```python
from build123d import *

# Parameters (mm, degrees)
F0_W     = 35
F0_H     = 15
F0_W_2   = 10
F0_R     = 2
F1_DEPTH = 6
F2_SIZE  = 3
F3_R     = 2
F4_DEPTH = 12
F5_DEPTH = 6
F6_R     = 2
F7_DEPTH = 15.001


with BuildPart() as f1:
    # F0 (on Top) → F1 (new body)
    with BuildSketch(Plane.XY):
        with Locations((22.5, 0)):
            Rectangle(F0_W, F0_H)
        Rectangle(F0_W_2, F0_H)
        Circle(F0_R, mode=Mode.SUBTRACT)
        with Locations((-22.5, 0)):
            Rectangle(F0_W, F0_H)
    extrude(amount=F1_DEPTH)

    # F2
    f2_edges = [f1.edges().sort_by_distance(p)[0] for p in [
        (0, -7.5, 6),
        (-40, 0, 6),
        (40, 0, 6),
        (0, 7.5, 6),
    ]]
    chamfer(f2_edges, length=F2_SIZE)

    # F3 (on face) → F4 (cut)
    with BuildSketch(Plane(origin=(0, 0, 0), x_dir=(1, 0, 0), z_dir=(0, 0, -1))):
        with Locations((-30, 0)):
            Circle(F3_R)
        with Locations((-15, 0)):
            Circle(F3_R)
        with Locations((15, 0)):
            Circle(F3_R)
        with Locations((30, 0)):
            Circle(F3_R)
    extrude(amount=-F4_DEPTH, mode=Mode.SUBTRACT)

    # F0 (on Top) → F5 (join)
    with BuildSketch(Plane.XY):
        Rectangle(F0_W_2, F0_H)
        Circle(F0_R, mode=Mode.SUBTRACT)
    extrude(amount=F5_DEPTH)

    # F6 (on face) → F7 (cut, through all)
    with BuildSketch(Plane.XZ.offset(7.5)):
        with Locations((0, 3)):
            Circle(F6_R)
    extrude(amount=-F7_DEPTH, mode=Mode.SUBTRACT)


solid = f1.part
```
The model under review builds one solid part; all positions refer to its coordinate system, in mm. A direction names the side the tool comes from. Give positions to 0.01 mm unless a question says otherwise; leave off trailing zeros. Write each loop counter-clockwise with the first axis right and the second up, starting at its lowest first coordinate (ties: lowest second). Pieces come first, ordered by that corner, then holes. Notation, with made-up numbers: (1.25, -40) - (6.25, -40) arc R23 cw to (6.25, -8) - close; hole circle Ø10 at (1.5, -32). An arc over 180 degrees is marked (long way). Answer in a Markdown table with one row per item. Add a question column.
1. We need section A-A on x = 0. Write out the cut boundary in (y, z), then the cut area to 3 significant figures.
2. Wall thickness on line 1 along X through (y, z) = (-0.75, 1.4); line 2 along X through (y, z) = (-5, 3); line 3 along X through (y, z) = (0, 3.35): over which ranges is each line inside the solid? List them lowest first. Write a range as [from, to].
3. We need section D-D on z = 4.1. Write out the cut boundary in (x, y).
4. Insertion check: P1, Ø3, axis at y = -5, z = 5, coming from the -X side; P2, Ø2.5, axis at x = 0, z = 3, coming from the -Y side; P3, Ø1.5, axis at y = 6.5, z = 4.5, coming from the +X side; P4, Ø0.9, axis at y = -6, z = 4.5, coming from the +X side. Each pin has a flat end and moves straight along its axis. Give the tip position at first contact, or say it passes through.
5. We need section B-B on x = -30. Write out the cut boundary in (y, z), then the cut area to 3 significant figures.
6. We need section C-C on y = 3.75. Write out the cut boundary in (x, z), then the cut area to 3 significant figures.
7. Draft analysis for pull direction Y (two halves, no side actions). For faces 5 (the cylindrical face through (-1.6, -4.6, 1.8)), 6 (the cylindrical face through (31.908, -0.601, 2.958)), 7 (the flat face through (1, 7.5, 1)), state which applies: +Y half, -Y half, draft (parallel to the pull), parting line (faces both ways), or undercut.
8. Tool access review of faces 1 (the flat face through (-5, 7, 5)), 2 (the cylindrical face through (-2, 0, 5)), 3 (the flat face through (5, 7, 5)), 4 (the flat face through (-22.7, -6, 4.5)): name each direction out of +Z, -Z, +X, -X, +Y, -Y from which nothing blocks a thin tool from reaching the whole face with its end or side.
Ans:
| question | item | result |
|---|---|---|
| 1 | outline | (-7.5, 0) - (-2, 0) - (-2, 1) - (-7.5, 1) - close; (-7.5, 5) - (-2, 5) - (-2, 6) - (-7.5, 6) - close; (2, 0) - (7.5, 0) - (7.5, 1) - (2, 1) - close; (2, 5) - (7.5, 5) - (7.5, 6) - (2, 6) - close |
| 1 | area | 22.0 mm^2 |
| 2 | line 1 | x = [-40, -31.85], [-28.15, -16.85], [-13.15, -1.85], [1.85, 13.15], [16.85, 28.15], [31.85, 40] |
| 2 | line 2 | x = [-40, -2], [2, 40] |
| 2 | line 3 | x = [-39.65, -32], [-28, -17], [-13, -2], [2, 13], [17, 28], [32, 39.65] |
| 3 | outline | (-38.9, -6.4) - (-5, -6.4) - (-5, -7.5) - (-1.67, -7.5) - (-1.67, -1.1) arc R2 cw to (-1.67, 1.1) - (-1.67, 7.5) - (-5, 7.5) - (-5, 6.4) - (-38.9, 6.4) - close; (1.67, -7.5) - (5, -7.5) - (5, -6.4) - (38.9, -6.4) - (38.9, 6.4) - (5, 6.4) - (5, 7.5) - (1.67, 7.5) - (1.67, 1.1) arc R2 cw to (1.67, -1.1) - close; hole circle Ø4 at (-30, 0); hole circle Ø4 at (-15, 0); hole circle Ø4 at (15, 0); hole circle Ø4 at (30, 0) |
| 4 | P1 | stops at x = -39.5 |
| 4 | P2 | passes through |
| 4 | P3 | stops at x = 39.25 |
| 4 | P4 | stops at x = 38.95 |
| 5 | outline | (-7.5, 0) - (-2, 0) - (-2, 6) - (-4.5, 6) - (-7.5, 3) - close; (2, 0) - (7.5, 0) - (7.5, 3) - (4.5, 6) - (2, 6) - close |
| 5 | area | 57.0 mm^2 |
| 6 | outline | (-40, 0) - (40, 0) - (40, 3) - (37, 6) - (-37, 6) - (-40, 3) - close; hole circle Ø4 at (0, 3) |
| 6 | area | 458 mm^2 |
| 7 | face 5 | draft |
| 7 | face 6 | undercut |
| 7 | face 7 | +Y half |
| 8 | face 1 | +Z, -X, +Y |
| 8 | face 2 | +Z, -Z |
| 8 | face 3 | +Z, +X, +Y |
| 8 | face 4 | +Z, -X, -Y |
